from build123d import *

# Parameters (mm, degrees)
F0_R     = 279.4
F0_R_2   = 171.45
F1_DEPTH = 241.3


with BuildPart() as f1:
    # F0 (on Front) → F1 (new body)
    with BuildSketch(Plane.XZ):
        Circle(F0_R)
        Circle(F0_R_2, mode=Mode.SUBTRACT)
    extrude(amount=F1_DEPTH)

    # F2 (on Top) → F3 (revolve, cut)
    with BuildSketch(Plane.XY):
        Polygon((-218.313, -213.36), (-218.313, -248.940435), (-138.143639, -248.940435), (-150.698322, -174.322647), (-162.82623, -167.260711), (-175.006, -188.356692), align=None)
    revolve(axis=Axis((0, -122.0978, 0), (0, -1, 0)), mode=Mode.SUBTRACT)


solid = f1.part
Could you check a few things on this model? Use its own coordinates, in mm. A direction names the side the tool comes from. Give positions to 0.01 mm unless a question says otherwise; leave off trailing zeros. Write each loop counter-clockwise with the first axis right and the second up, starting at its lowest first coordinate (ties: lowest second). Pieces come first, ordered by that corner, then holes. Notation, with made-up numbers: (-17, -37) -> (30, -37) arc R11 ccw to (30, -21) -> close; hole circle Ø7 at (-23, -25.75). An arc over 180 degrees is marked (long way). Answer as CSV lines item,"result". Start each with the question number.
(1) If we section it at C-C, the plane y = -93: Write out the boundary of the cut face in (x, z).
(2) If we mould it in two halves opening along Z, with no side actions, what happens to faces 1 (the face through (-221.722, -118.961, -170.011)), 2 (the face through (120, 0, 128)), 3 (the face through (136.23, -182.58, 104.46))? For each: +Z half, -Z half, draft (parallel to the pull), parting line (faces both ways), or undercut.
(3) If we section it at A-A, the plane z = 0: Write out the boundary of the cut face in (x, y), and give its area (3 significant figures).
(4) Please list where these lines run through material, in increasing order: line 1 (Z direction, x = 0, y = -67); line 2 (X direction, y = -112, z = 16.5); line 3 (X direction, y = -157, z = -134).
(5) Which directions (+Z, -Z, +X, -X, +Y, -Y) give clear straight access to the entire face, cutting with the end or side of a thin tool? Please do faces 4 (the face through (-167, -241.3, -144)), 5 (the face through (47.33, -227.53, 213.12)).
(6) If we section it at B-B, the plane x = 0: Write out the boundary of the cut face in (y, z).
(7) I'm going to push flat-ended pins straight in: pin 1 Ø3 at (y, z) = (-67.5, 218) entering from +X; pin 2 Ø1 at (y, z) = (-129.5, 112) entering from -X; pin 3 Ø5 at (x, y) = (216.5, -182.5) entering from -Z. Where does each tip first touch, or does it pass through?
Answer list:
1,outline,"circle Ø558.8 at (0, 0); hole circle Ø342.9 at (0, 0)"
2,face 1,"parting line"
2,face 2,"draft"
2,face 3,"undercut"
3,outline,"(-279.4, -241.3) -> (-218.31, -241.3) -> (-218.31, -213.36) -> (-175.01, -188.36) -> (-171.45, -182.2) -> (-171.45, 0) -> (-279.4, 0) -> close; (171.45, -182.2) -> (175.01, -188.36) -> (218.31, -213.36) -> (218.31, -241.3) -> (279.4, -241.3) -> (279.4, 0) -> (171.45, 0) -> close"
3,area,"48,200 mm^2"
4,line 1,"-279.4 to -171.45, 171.45 to 279.4"
4,line 2,"-278.91 to -170.65, 170.65 to 278.91"
4,line 3,"-245.17 to -106.95, 106.95 to 245.17"
5,face 4,"+Z, -Z, +X, -X, -Y"
5,face 5,"-Y"
6,outline,"(-241.3, -279.4) -> (0, -279.4) -> (0, -171.45) -> (-182.2, -171.45) -> (-188.36, -175.01) -> (-213.36, -218.31) -> (-241.3, -218.31) -> close; (-241.3, 218.31) -> (-213.36, 218.31) -> (-188.36, 175.01) -> (-182.2, 171.45) -> (0, 171.45) -> (0, 279.4) -> (-241.3, 279.4) -> close"
7,pin 1,"x = 176.61"
7,pin 2,"x = -256.19"
7,pin 3,"z = -179.63"
